from build123d import *

# Parameters (mm, degrees)
PAD008_DEPTH       = 2
SKETCH037_R        = 3
PAD009_DEPTH       = 21
SKETCH038_R        = 1.6
POCKET003005_DEPTH = 30


with BuildPart() as part:
    # Sketch035 → Pad008 (new body)
    with BuildSketch(Plane.XY):
        with BuildLine():
            Line((24.97547, -25.036306), (-25.000607, -25.036306))
            ThreePointArc((-28.013759, -22.023154), (-27.131227, -24.153774), (-25.000607, -25.036306))
            Line((-28.013759, -22.023154), (-28.013759, 37.989404))
            ThreePointArc((-25.000624, 41.000002), (-27.131078, 40.119115), (-28.013759, 37.989404))
            Line((-25.000624, 41.000002), (-9.513229, 41.000002))
            ThreePointArc((-7.513229, 39.000002), (-8.099015, 40.414215), (-9.513229, 41.000002))
            Line((-7.513229, 26), (-7.513229, 39.000002))
            ThreePointArc((-7.513229, 26), (-6.927443, 24.585787), (-5.513229, 24))
            Line((5.476271, 24), (-5.513229, 24))
            ThreePointArc((5.476271, 24), (6.890485, 24.585787), (7.476271, 26))
            Line((7.476271, 39.000016), (7.476271, 26))
            ThreePointArc((9.476271, 41.000016), (8.062057, 40.41423), (7.476271, 39.000016))
            Line((9.476271, 41.000016), (24.999953, 41.000016))
            ThreePointArc((28, 38.041338), (27.106731, 40.135916), (24.999953, 41.000016))
            Line((28, 38.041338), (28, 37))
            ThreePointArc((25, 34), (27.12132, 34.87868), (28, 37))
            Line((25, 34), (22, 34))
            ThreePointArc((22, 34), (21.292893, 33.707107), (21, 33))
            Line((21, -16), (21, 33))
            ThreePointArc((21, -16), (21.292893, -16.707107), (22, -17))
            Line((25, -17), (22, -17))
            ThreePointArc((27.999984, -19.999984), (27.121309, -17.878675), (25, -17))
            Line((27.999984, -22.011792), (27.999984, -19.999984))
            ThreePointArc((24.97547, -25.036306), (27.114124, -24.150446), (27.999984, -22.011792))
        make_face()
    extrude(amount=-PAD008_DEPTH)

    # Sketch037 → Pad009 (join)
    with BuildSketch(Plane(origin=(0, 0, -2), x_dir=(1, 0, 0), z_dir=(0, 0, -1))):
        with Locations((-24.440964, 20.497406)):
            Circle(SKETCH037_R)
        with Locations((24.491911, 20.496445)):
            Circle(SKETCH037_R)
        with Locations((-24.511511, -37.516029)):
            Circle(SKETCH037_R)
        with Locations((24.504074, -37.505135)):
            Circle(SKETCH037_R)
    extrude(amount=PAD009_DEPTH)

    # Sketch038 (on Face31 of Pad009) → Pocket003005 (cut)
    with BuildSketch(Plane(origin=(0, 0, -23), x_dir=(1, 0, 0), z_dir=(0, 0, -1))):
        with Locations((-24.440964, 20.497406)):
            Circle(SKETCH038_R)
        with Locations((24.491911, 20.496445)):
            Circle(SKETCH038_R)
        with Locations((-24.511511, -37.516029)):
            Circle(SKETCH038_R)
        with Locations((24.504074, -37.505135)):
            Circle(SKETCH038_R)
    extrude(amount=-POCKET003005_DEPTH, mode=Mode.SUBTRACT)


with BuildPart() as part_1:
    # Body007 placement: moved
    add(part.part.moved(Location((0, 0, 23))))


solid = part_1.part
Verification items for the finished model (mm, model axes). A direction names the side the tool comes from. Give positions to 0.01 mm unless a question says otherwise; leave off trailing zeros. Write each loop counter-clockwise with the first axis right and the second up, starting at its lowest first coordinate (ties: lowest second). Pieces come first, ordered by that corner, then holes. Notation, with made-up numbers: (70, 6) -> (122, 6) arc R26 cw to (122, 39) -> close; hole circle Ø9 at (-16.5, 19). An arc over 180 degrees is marked (long way). Use CSV: the item, a comma, the result in double quotes.
(1) Set-up check for faces 4 (the cylindrical face through (-22.83, -23.03, 10.65)), 5 (the flat face through (26, -19, 0)), 6 (the flat face through (0, 24, 22)), 7 (the cylindrical face through (23.325, 36.424, 11.339)), 8 (the flat face through (24, -17, 22)): record each of +Z, -Z, +X, -X, +Y, -Y from which the full face is reachable in a straight line by a thin tool's end or side.
Derived:
face 4,"-Z"
face 5,"-Z, +X, -X, +Y, -Y"
face 6,"+Z, -Z, +Y"
face 7,"+Z, -Z"
face 8,"+Z, -Z, +X"
(2) Sectioned sample at B-B (y = 25). Record the cut outline in (x, z).
Derived:
outline,"(-28.01, 21) -> (-7.25, 21) -> (-7.25, 23) -> (-28.01, 23) -> close; (7.21, 21) -> (21, 21) -> (21, 23) -> (7.21, 23) -> close"
(3) Material ranges on L1, parallel to X at y = -20.5, z = 6.25; L2, parallel to X at y = 37, z = 15.75; L3, parallel to Z at x = -14, y = 16.5, recorded low to high.
Derived:
L1,"x = -27.44 to -26.04, -22.84 to -21.44, 21.49 to 22.89, 26.09 to 27.49"
L2,"x = -27.47 to -26.03, -23 to -21.56, 21.55 to 22.99, 26.02 to 27.46"
L3,"z = 21 to 23"
(4) Sectioned sample at A-A (z = 20). Record the cut outline in (x, y).
Derived:
outline,"circle Ø6 at (-24.51, 37.52); circle Ø6 at (-24.44, -20.5); circle Ø6 at (24.49, -20.5); circle Ø6 at (24.5, 37.51); hole circle Ø3.2 at (-24.51, 37.52); hole circle Ø3.2 at (-24.44, -20.5); hole circle Ø3.2 at (24.49, -20.5); hole circle Ø3.2 at (24.5, 37.51)"
(5) Sectioned sample at D-D (x = 2.5). Record the cut outline in (y, z).
Derived:
outline,"(-25.04, 21) -> (24, 21) -> (24, 23) -> (-25.04, 23) -> close"
(6) Sectioned sample at C-C (y = 15). Record the cut outline in (x, z).
Derived:
outline,"(-28.01, 21) -> (21, 21) -> (21, 23) -> (-28.01, 23) -> close"
(7) Go/stop test with flat-tipped pins: pin 1 (1 mm diameter, centred on y = 4.5, z = 22, fed in from +X); pin 2 (1.5 mm diameter, centred on x = 0.5, y = 23.5, fed in from -Z); pin 3 (3 mm diameter, centred on x = -24.51, y = 37.52, fed in from -Z); pin 4 (4 mm diameter, centred on x = -24.44, y = -20.5, fed in from +Z). Record where each tip stops, or that it passes through.
Derived:
pin 1,"stops at x = 21"
pin 2,"stops at z = 21"
pin 3,"passes through"
pin 4,"stops at z = 23"
(8) Release check for a two-part mould opening along X. For faces 1 (the flat face through (17, 41, 22)), 2 (the cylindrical face through (27.09, -24.174, 22.014)), 3 (the flat face through (-7.513, 32, 22)) record: +X half, -X half, draft (parallel to the pull), parting line (faces both ways), or undercut.
Derived:
face 1,"draft"
face 2,"+X half"
face 3,"undercut"
